Design review of the part built by this model. Coordinates are the model's own, in mm. A direction names the side the tool comes from. Coordinates: 2 decimals unless noted, no trailing zeros. Write each loop counter-clockwise with the first axis right and the second up, starting at its lowest first coordinate (ties: lowest second). Pieces come first, ordered by that corner, then holes.
```python
from build123d import *

# Parameters (mm, degrees)
SKETCH_1_W          = 12
SKETCH_1_H          = 12
SKETCH_1_W_2        = 8
SKETCH_1_H_2        = 8
EXTRUDE_1_DEPTH     = 200
CUT_EXTRUDE_1_DEPTH = 12
CUT_EXTRUDE_3_DEPTH = 200
SKETCH_6_R          = 1
CUT_EXTRUDE_4_DEPTH = 12
SKETCH_7_R          = 1
CUT_EXTRUDE_5_DEPTH = 12


with BuildPart() as part:
    # 草图1 → 凸台-拉伸1 (new body)
    with BuildSketch(Plane(origin=(0, 0, 0), x_dir=(1, 0, 0), z_dir=(0, 1, 0))):
        with Locations((6, 6)):
            Rectangle(SKETCH_1_W, SKETCH_1_H)
        with Locations((6, 6)):
            Rectangle(SKETCH_1_W_2, SKETCH_1_H_2, mode=Mode.SUBTRACT)
    extrude(amount=EXTRUDE_1_DEPTH)

    # 草图2 → 切除-拉伸1 (cut)
    with BuildSketch(Plane.ZY):
        with BuildLine():
            ThreePointArc((-7, 190), (-6, 189), (-5, 190))
            Line((-5, 190), (-7, 190))
        make_face()
        with BuildLine():
            Line((-7, 190), (-5, 190))
            ThreePointArc((-5, 190), (-6, 191), (-7, 190))
        make_face()
    extrude(amount=-CUT_EXTRUDE_1_DEPTH, mode=Mode.SUBTRACT)

    # 草图4 → 切除-拉伸3 (cut)
    with BuildSketch(Plane(origin=(0, 0, 0), x_dir=(-1, 0, 0), z_dir=(0, -1, 0))):
        Polygon((-11, 6), (-11, 1), (-1, 1), (-1, 11), (-11, 11), align=None)
    extrude(amount=-CUT_EXTRUDE_3_DEPTH, mode=Mode.SUBTRACT)

    # 草图6 → 切除-拉伸4 (cut)
    with BuildSketch(Plane(origin=(12, 0, 0), x_dir=(0, 0, -1), z_dir=(1, 0, 0))):
        with Locations((6, 5)):
            Circle(SKETCH_6_R)
    extrude(amount=-CUT_EXTRUDE_4_DEPTH, mode=Mode.SUBTRACT)

    # 草图7 → 切除-拉伸5 (cut)
    with BuildSketch(Plane.ZY):
        with Locations((-6, 50)):
            Circle(SKETCH_7_R)
    extrude(amount=-CUT_EXTRUDE_5_DEPTH, mode=Mode.SUBTRACT)


solid = part.part
```
(1) Consider section C-C (y = 77). Give the boundary of the cut face in (x, z), plus the area to 3 significant figures.
(2) Mouldability with a two-part tool opening along X and no side actions: class faces 1 (the flat face through (11, 99, -6)), 2 (the flat face through (12, 99, -6)), 3 (the flat face through (0, 99, -6)) as +X half, -X half, draft (parallel to the pull), parting line (faces both ways), or undercut.
(3) Consider section A-A (x = 7.5). Give the boundary of the cut face in (y, z), plus the area to 3 significant figures.
(4) Wall thickness on line 1 (Y direction, x = 0.4, z = -6); line 2 (Z direction, x = 7.5, y = 20); line 3 (X direction, y = 84, z = -9.5): over which ranges is each line inside the solid? List them lowest first.
(5) Consider section B-B (z = -9.25). Give the boundary of the cut face in (x, y), plus the area to 3 significant figures.
(6) Insertion check: pin 1 Ø5 at (x, y) = (3.5, 78.5) entering from +Z. The pin has a flat end and moves straight along its axis. Give the tip position at first contact, or say it passes through.
(7) For faces 4 (the flat face through (11.2, 200, -6.1)), 5 (the flat face through (6, 99, -11)), list the 3-axis set-ups (+Z, -Z, +X, -X, +Y, -Y) from which the entire face can be reached by the end or side of a thin tool; tool diameter is ignored.
Results:
1. outline: (0, -12) - (12, -12) - (12, 0) - (0, 0) - close; hole (1, -11) - (11, -11) - (11, -1) - (1, -1) - close
1. area: 44.0 mm2
2. face 1: undercut
2. face 2: +X half
2. face 3: -X half
3. outline: (0, -12) - (200, -12) - (200, -11) - (0, -11) - close; (0, -1) - (200, -1) - (200, 0) - (0, 0) - close
3. area: 400 mm2
4. line 1: y = 0 to 4, 6 to 49, 51 to 189, 191 to 200
4. line 2: z = -12 to -11, -1 to 0
4. line 3: x = 0 to 1, 11 to 12
5. outline: (0, 0) - (1, 0) - (1, 200) - (0, 200) - close; (11, 0) - (12, 0) - (12, 200) - (11, 200) - close
5. area: 400 mm2
6. pin 1: stops at z = 0
7. face 4: +Z, -Z, +X, -X, +Y
7. face 5: +Y, -Y
